```python
from build123d import *

# Parameters (mm, degrees)
F1_DEPTH = 3
F0_R     = 2.25
F2_DEPTH = 8
F3_SIZE  = 1.5
F4_SIZE  = 2


with BuildPart() as f1:
    # F0 (on Front) → F1 (new body)
    with BuildSketch(Plane.XZ):
        Polygon((-20, -5), (-20, 0), (-34, 0), (-34, -10), (33, -9), (33, 0), (20, 0), (20, -5), align=None)
    extrude(amount=F1_DEPTH)

    # F0 (on Front) → F2 (join)
    with BuildSketch(Plane.XZ):
        Polygon((20, 5), (-20, 5), (-20, 0), (-20, -5), (20, -5), (20, 0), align=None)
        with Locations((-10, 0)):
            Circle(F0_R, mode=Mode.SUBTRACT)
        with Locations((10, 0)):
            Circle(F0_R, mode=Mode.SUBTRACT)
    extrude(amount=F2_DEPTH)

    # F3
    f3_edges = [f1.edges().sort_by_distance(p)[0] for p in [
        (7.75, 0, 0),
        (-12.25, 0, 0),
    ]]
    chamfer(f3_edges, length=F3_SIZE)

    # F4
    f4_edges = [f1.edges().sort_by_distance(p)[0] for p in [
        (-27, -3, 0),
        (26.5, -3, 0),
    ]]
    chamfer(f4_edges, length=F4_SIZE)


solid = f1.part
```
Source: CAD feature listing. Evaluate the final solid. Frame: model axes, mm. A direction names the side the tool comes from. Round coordinates to 2 decimals unless told otherwise and drop trailing zeros. Loops run counter-clockwise (first coordinate to the right, second up) from the corner with the lowest first, then second, coordinate; pieces in that order, holes last. Notation, with made-up numbers: M 44.5,-34 L 66.5,-34 A28 cw 66.5,-7 Z; hole C 18.5,81 d10. An arc over 180 degrees is marked long. Use a Markdown table: item, result. Add a question column.
1. Contact query for flat-ended pins moving along their axis: pin 1 (1.5 mm diameter, centred on x = -7, y = -1, fed in from -Z); pin 2 (4 mm diameter, centred on y = -4.5, z = -2, fed in from +X); pin 3 (5 mm diameter, centred on x = 10, z = 0, fed in from +Y); pin 4 (0.8 mm diameter, centred on x = -27, y = -0.5, fed in from +Z). Output: stop coordinate, or through.
2. Cut plane B-B, the plane x = -10. Output: boundary loops of the cut face in (y, z), and give its area (3 significant figures).
3. Ray query, line 1 along Z through (x, y) = (-10, -4); line 2 along X through (y, z) = (-1, 0.25); line 3 along X through (y, z) = (-2.75, 1). Return the intervals inside material, ascending. Write a range as [from, to].
4. Cut plane A-A, the plane y = -2.25. Output: boundary loops of the cut face in (x, z).
5. Pull-direction query (Z, two-part tool) for faces 4 (the flat face through (0, -5, -5)), 5 (the flat face through (27, -2, -1)), 6 (the cylindrical face through (-12.248, -4.704, 0.099)), 7 (the flat face through (33, -1, -5)); classes: +Z half, -Z half, draft (parallel to the pull), parting line (faces both ways), or undercut.
6. Cut plane C-C, the plane z = -8. Output: boundary loops of the cut face in (x, y), and give its area (3 significant figures).
7. Cut plane D-D, the plane x = 2.5. Output: boundary loops of the cut face in (y, z).
8. Set-up query: faces 1 (the cylindrical face through (7.752, -4.704, 0.099)), 2 (the flat face through (-20, -4, 0)), 3 (the flat face through (20, -5, 0)). Return all of +Z, -Z, +X, -X, +Y, -Y with unobstructed straight access to the full face (end or side cutting, diameter ignored); none if empty.
Solution:
| question | item | result |
|---|---|---|
| 1 | pin 1 | stops at z = -9.61 |
| 1 | pin 2 | stops at x = 33 |
| 1 | pin 3 | stops at y = -1.25 |
| 1 | pin 4 | stops at z = 0 |
| 2 | outline | M -8,-5 L -3,-5 L -3,-9.64 L 0,-9.64 L 0,-3.75 L -1.5,-2.25 L -8,-2.25 Z; M -8,2.25 L -1.5,2.25 L 0,3.75 L 0,5 L -8,5 Z |
| 2 | area | 55.7 mm2 |
| 3 | line 1 | z = [-5, -2.25], [2.25, 5] |
| 3 | line 2 | x = [-20, -12.74], [-7.26, 7.26], [12.74, 20] |
| 3 | line 3 | x = [-20, -12.02], [-7.98, 7.98], [12.02, 20] |
| 4 | outline | M -34,-10 L 33,-9 L 33,-1.25 L 20,-1.25 L 20,5 L -20,5 L -20,-1.25 L -34,-1.25 Z; hole C -10,0 d4.5; hole C 10,0 d4.5 |
| 5 | face 4 | -Z half |
| 5 | face 5 | +Z half |
| 5 | face 6 | undercut |
| 5 | face 7 | draft |
| 6 | outline | M -34,-3 L 33,-3 L 33,0 L -34,0 Z |
| 6 | area | 201 mm2 |
| 7 | outline | M -8,-5 L -3,-5 L -3,-9.46 L 0,-9.46 L 0,5 L -8,5 Z |
| 8 | face 1 | +Y, -Y |
| 8 | face 2 | +Z, -X, -Y |
| 8 | face 3 | +Z, +X, -Y |
